The listing builds one solid part. Answer for the finished solid, in the listing's coordinates (mm). Face numbers are marked on the shaded views. A direction names the side the tool comes from. Give positions to 0.01 mm unless a question says otherwise; leave off trailing zeros. Order: outer loops, then holes, each group sorted by start corner. A loop starts at its lowest first (then second) coordinate and runs counter-clockwise, first axis right, second up. Notation, with made-up numbers: (-20, 58.25) - (-4, 58.25) arc R22 cw to (-4, 80.25) - close; hole circle Ø4 at (31.5, 24.25). An arc over 180 degrees is marked (long way). Answer in a Markdown table with one row per item. Add a question column.
```python
from build123d import *

# Parameters (mm, degrees)
F0_W     = 31.75
F0_H     = 9.525
F1_DEPTH = 3.175
F4_R     = 2.286
F8_R     = 2.286


with BuildPart() as f1:
    # F0 (on Top) → F1 (new body)
    with BuildSketch(Plane.XY):
        with Locations((15.875, 4.7625)):
            Rectangle(F0_W, F0_H)
    extrude(amount=F1_DEPTH)

    # F5: sweep along a path in F3
    with BuildLine(Plane.YZ.offset(28.575)) as f5_path:
        Line((7.1374, 3.175), (7.1374, 9.525))
        Line((7.1374, 9.525), (11.6275280605, 14.0151280605))
    # F4 (on face) → F5 (sweep)
    with BuildSketch(Plane.XY.offset(3.175)):
        with Locations((28.575, 7.1374)):
            Circle(F4_R)
    sweep(path=f5_path.line, transition=Transition.RIGHT)

    # F9: sweep along a path in F7
    with BuildLine(Plane.YZ.offset(3.175)) as f9_path:
        Line((7.1374, 3.175), (7.1374, 9.525))
        Line((7.1374, 9.525), (11.6275280605, 14.0151280605))
    # F8 (on face) → F9 (sweep)
    with BuildSketch(Plane.XY.offset(3.175)):
        with Locations((3.175, 7.1374)):
            Circle(F8_R)
    sweep(path=f9_path.line, transition=Transition.RIGHT)


solid = f1.part
```
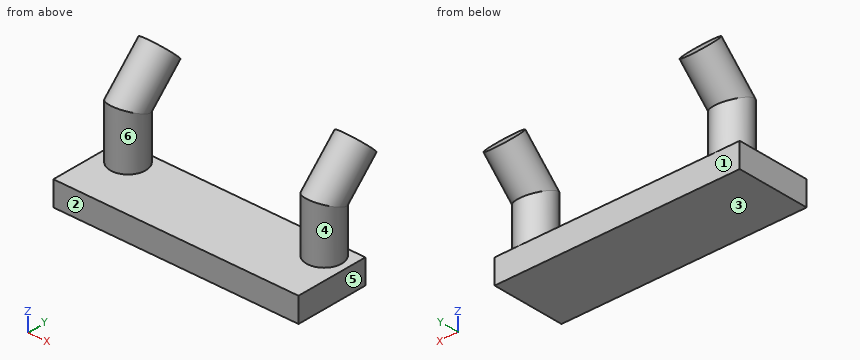
(1) Each of these flat-tipped pins is pushed along its axis until it touches: P1, Ø4, axis at y = 4, z = 9, coming from the -X side; P2, Ø3, axis at y = 11.5, z = 14, coming from the -X side; P3, Ø2, axis at x = 28, z = 5.5, coming from the +Y side. Where does it stop, or does it pass through?
(2) The mould has two halves that part along Z. Classify the marked faces 3, 4, 5 and 6: +Z half, -Z half, draft (parallel to the pull), parting line (faces both ways), or undercut.
(3) Straight lines are drawn through the part: line 1 (Z direction, x = 7.5, y = 1.5) (3 decimals); line 2 (X direction, y = 7, z = 12); line 3 (X direction, y = 9.5, z = 11.5). For each, find the intervals that lie inside material, in ascending order.
(4) Find section A-A, the plane x = 27. Write down the section's boundary in (y, z) (3 decimals).
(5) Find section B-B, the plane y = 1.5. Write down the section's boundary in (x, z) (3 decimals), plus the area to 3 significant figures.
(6) Find section C-C, the plane z = 2.5. Write down the section's boundary in (x, y) (3 decimals).
(7) For the marked faces 1 and 2, determine the directions among +Z, -Z, +X, -X, +Y, -Y from which every point of the face is accessible in a straight line to the end or side of a thin tool.
Answer key:
| question | item | result |
|---|---|---|
| 1 | P1 | x = 1.19 |
| 1 | P2 | x = 0.89 |
| 1 | P3 | y = 9.42 |
| 2 | face 3 | -Z half |
| 2 | face 4 | undercut |
| 2 | face 5 | draft |
| 2 | face 6 | undercut |
| 3 | line 1 | 0 to 3.175 |
| 3 | line 2 | 1.83 to 4.52, 27.23 to 29.92 |
| 3 | line 3 | 0.91 to 5.44, 26.31 to 30.84 |
| 4 | outline | (0, 0) - (9.525, 0) - (9.525, 3.175) - (8.794, 3.175) - (8.794, 8.839) - (12.799, 12.844) - (10.456, 15.187) - (5.481, 10.211) - (5.481, 3.175) - (0, 3.175) - close |
| 5 | outline | (0, 0) - (31.75, 0) - (31.75, 3.175) - (0, 3.175) - close |
| 5 | area | 101 mm² |
| 6 | outline | (0, 0) - (31.75, 0) - (31.75, 9.525) - (0, 9.525) - close |
| 7 | face 1 | -Z, +X, -X, +Y |
| 7 | face 2 | +Z, -Z, +X, -X, -Y |
